```python
from build123d import *

# Parameters (mm, degrees)
BOSS_EXTRUDE1_DEPTH = 2
SKETCH2_R           = 1.571161349
CUT_EXTRUDE1_DEPTH  = 2
CHAMFER1_SIZE       = 0.5
SKETCH4_W           = 2
SKETCH4_H           = 12.352861416
CUT_EXTRUDE2_DEPTH  = 13.5
SKETCH5_R           = 1
CUT_EXTRUDE3_DEPTH  = 13.5
SKETCH6_R           = 3
BOSS_EXTRUDE2_DEPTH = 1
CHAMFER2_SIZE       = 0.2


with BuildPart() as part:
    # Sketch1 → Boss-Extrude1 (new body)
    with BuildSketch(Plane.XY):
        with BuildLine():
            Line((-6.32455532, 9), (6.32455532, 9))
            ThreePointArc((6.32455532, 9), (11, 0), (6.32455532, -9))
            Line((6.32455532, -9), (-6.32455532, -9))
            ThreePointArc((-6.32455532, -9), (-11, 0), (-6.32455532, 9))
        make_face()
    extrude(amount=BOSS_EXTRUDE1_DEPTH)

    # Sketch2 → Cut-Extrude1 (cut)
    with BuildSketch(Plane.XY.offset(2)):
        with Locations((4.949747468, 4.949747468)):
            Circle(SKETCH2_R)
        with Locations((4.949747468, -4.949747468)):
            Circle(SKETCH2_R)
        with Locations((-4.949747468, -4.949747468)):
            Circle(SKETCH2_R)
        with Locations((-4.949747468, 4.949747468)):
            Circle(SKETCH2_R)
    extrude(amount=-CUT_EXTRUDE1_DEPTH, mode=Mode.SUBTRACT)

    # Chamfer1
    chamfer1_edges = [part.edges().sort_by_distance(p)[0] for p in [
        (-6.520908817, 4.949747468, 0),
        (-6.520908817, -4.949747468, 0),
        (3.378586119, -4.949747468, 0),
        (3.378586119, 4.949747468, 0),
    ]]
    chamfer(chamfer1_edges, length=CHAMFER1_SIZE)

    # Sketch3 → Revolve1 (revolve)
    with BuildSketch(Plane(origin=(0, 0, 0), x_dir=(1, 0, 0), z_dir=(0, 1, 0))):
        with BuildLine():
            Line((0, 0), (0, 14))
            ThreePointArc((0, 14), (2.828427125, 12.828427125), (4, 10))
            Line((4, 10), (4, 0))
            Line((4, 0), (0, 0))
        make_face()
    revolve(axis=Axis((0, 0, 0), (0, 0, -1)))

    # Sketch4 → Cut-Extrude2 (cut, symmetric)
    with BuildSketch(Plane(origin=(0, 0, 0), x_dir=(1, 0, 0), z_dir=(0, 1, 0))):
        with Locations((0, 9.676430708)):
            Rectangle(SKETCH4_W, SKETCH4_H)
    extrude(amount=CUT_EXTRUDE2_DEPTH, both=True, mode=Mode.SUBTRACT)

    # Sketch5 → Cut-Extrude3 (cut, symmetric)
    with BuildSketch(Plane(origin=(0, 0, 0), x_dir=(0, 0, -1), z_dir=(1, 0, 0))):
        with Locations((8, 0)):
            Circle(SKETCH5_R)
    extrude(amount=CUT_EXTRUDE3_DEPTH, both=True, mode=Mode.SUBTRACT)

    # Sketch6 → Boss-Extrude2 (add)
    with BuildSketch(Plane.XY.offset(2)):
        Circle(SKETCH6_R)
    extrude(amount=BOSS_EXTRUDE2_DEPTH)

    # Chamfer2
    chamfer2_edges = [part.edges().sort_by_distance(p)[0] for p in [
        (-3, 0, 3),
    ]]
    chamfer(chamfer2_edges, length=CHAMFER2_SIZE)


solid = part.part
```
Check sheet for the modelled part. Datum: model origin and axes. Units: mm. A direction names the side the tool comes from. Coordinates: 2 decimals unless noted, no trailing zeros. Loops run counter-clockwise (first coordinate to the right, second up) from the corner with the lowest first, then second, coordinate; pieces in that order, holes last. Notation, with made-up numbers: M -12.75,30.5 L 23.25,30.5 A28 ccw 23.25,66.5 Z; hole C 75.5,72 d11. An arc over 180 degrees is marked long. Answer as a JSON object with one key per item and string values.
1. Sectioned sample at A-A on y = 0. Record the cut outline in (x, z).
Outcome:
{"outline": "M -11,0 L -4,0 L -4,-7 L -1,-7 L -1,-3.5 L 1,-3.5 L 1,-7 L 4,-7 L 4,0 L 11,0 L 11,2 L 3,2 L 3,2.8 L 2.8,3 L -2.8,3 L -3,2.8 L -3,2 L -11,2 Z; M -4,-10 A4 ccw -1,-13.87 L -1,-9 L -4,-9 Z; M 1,-13.87 A4 ccw 4,-10 L 4,-9 L 1,-9 Z"}
2. Sectioned sample at B-B on z = -7.5. Record the cut outline in (x, y).
Outcome:
{"outline": "M -3.91,-0.87 A4 ccw -1,-3.87 L -1,-0.87 Z; M -3.91,0.87 L -1,0.87 L -1,3.87 A4 ccw Z; M 1,-3.87 A4 ccw 3.91,-0.87 L 1,-0.87 Z; M 1,0.87 L 3.91,0.87 A4 ccw 1,3.87 Z"}
3. Scan lines: L1, parallel to Z at x = 8, y = -1.75; L2, parallel to X at y = -4, z = 1.75; L3, parallel to X at y = 0.75, z = -13. Record each from-to range of solid material in increasing order. Write a range as from..to.
Outcome:
{"L1": "0..2", "L2": "-10.25..-6.2, -3.7..3.7, 6.2..10.25", "L3": "-2.54..-1, 1..2.54"}
4. Access from +Z, -Z, +X, -X, +Y, -Y to the whole of each face (thin tool, end or side, straight path). Record for faces 1 (the cylindrical face through (-11, 0, 1)), 2 (the cylindrical face through (3.695, 1.532, -4.93)).
Outcome:
{"face 1": "+Z, -Z, -X", "face 2": "-Z"}
5. Sectioned sample at D-D on z = -11.75. Record the cut outline in (x, y), and give its area (3 significant figures).
Outcome:
{"outline": "M -1,-3.46 L -1,3.46 A3.6 ccw Z; M 1,-3.46 A3.6 ccw 1,3.46 Z", "area": "26.4 mm²"}
6. Depth check by flat-ended pin: P1, Ø5.5, axis at x = -3.5, y = -0.5, coming from the -Z side; P2, Ø1.5, axis at x = -2, z = -12, coming from the -Y side; P3, Ø4, axis at x = 4.95, y = 4.95, coming from the -Z side; P4, Ø1.6, axis at x = 0, y = -1, coming from the -Z side. Enter the tip coordinate at first touch or a pass-through.
Outcome:
{"P1": "z = -13.87", "P2": "y = -3.42", "P3": "z = 0.07", "P4": "z = -3.5"}
7. Sectioned sample at C-C on x = 0. Record the cut outline in (y, z).
Outcome:
{"outline": "M -9,0 L -4,0 L -4,-3.5 L 4,-3.5 L 4,0 L 9,0 L 9,2 L 3,2 L 3,2.8 L 2.8,3 L -2.8,3 L -3,2.8 L -3,2 L -9,2 Z"}
8. Release check for a two-part mould opening along Z. For faces 3 (the flat face through (-1, 1, -9)), 4 (the flat face through (0, 0, -3.5)), 5 (the cylindrical face through (-2.5, -0.6, -7.2)) record: pulls with the +Z half, pulls with the -Z half, needs draft (parallel to the pull), parting line crosses it, or undercut.
Outcome:
{"face 3": "needs draft", "face 4": "pulls with the -Z half", "face 5": "undercut"}
